```python
from build123d import *

# Parameters (mm, degrees)
BOSS_EXTRUDE1_DEPTH = 3


with BuildPart() as part:
    # Sketch1 → Boss-Extrude1 (new body)
    with BuildSketch(Plane(origin=(0, 0, 0), x_dir=(1, 0, 0), z_dir=(0, 1, 0))):
        with BuildLine():
            Line((0, 0), (3.5, 0))
            Line((3.5, 0), (3.5, 20))
            ThreePointArc((3.5, 20), (9.5, 26), (15.5, 20))
            ThreePointArc((15.5, 20), (17.25, 18.25), (19, 20))
            ThreePointArc((19, 20), (9.5, 29.5), (0, 20))
            Line((0, 20), (0, 0))
        make_face()
    extrude(amount=BOSS_EXTRUDE1_DEPTH)


solid = part.part
```
The model under review builds one solid part; all positions refer to its coordinate system, in mm. Round coordinates to 2 decimals unless told otherwise and drop trailing zeros. Loops run counter-clockwise (first coordinate to the right, second up) from the corner with the lowest first, then second, coordinate; pieces in that order, holes last. Notation, with made-up numbers: M 38,-24 L 49,-24 A26 cw 49,-3 Z; hole C -8.75,15.5 d3. An arc over 180 degrees is marked long. Put each result on its own line as item: value.
Q1. Consider section C-C, the plane x = 9.5. Give the boundary of the cut face in (y, z), then the cut area to 3 significant figures.
Result set:
outline: M 0,-29.5 L 3,-29.5 L 3,-26 L 0,-26 Z
area: 10.5 mm²
Q2. For pin 1 (10 mm diameter, centred on x = 3.5, z = -13, fed in from -Y), flat-tipped, find the tip position at first contact; note if it passes through.
Result set:
pin 1: stops at y = 0
Q3. Mouldability with a two-part tool opening along X and no side actions: class faces 1 (the cylindrical face through (17.21, 1.48, -18.25)), 2 (the cylindrical face through (9.709, 1.479, -29.498)), 3 (the flat face through (3, 3, -18)) as released by +X, released by -X, zero draft, split by the parting line, or undercut.
Result set:
face 1: undercut
face 2: split by the parting line
face 3: zero draft
Q4. Consider section B-B, the plane y = 0.7. Give the boundary of the cut face in (x, z), then the cut area to 3 significant figures.
Result set:
outline: M 0,-20 A9.5 ccw 19,-20 A1.75 ccw 15.5,-20 A6 cw 3.5,-20 L 3.5,0 L 0,0 Z
area: 160 mm²
Q5. Consider section A-A, the plane z = -19.25. Give the boundary of the cut face in (x, y).
Result set:
outline: M 0,0 L 3.5,0 L 3.5,3 L 0,3 Z; M 15.67,0 L 18.83,0 L 18.83,3 L 15.67,3 Z
Q6. Consider section D-D, the plane z = -3.5. Give the boundary of the cut face in (x, y), then the cut area to 3 significant figures.
Result set:
outline: M 0,0 L 3.5,0 L 3.5,3 L 0,3 Z
area: 10.5 mm²
Q7. To check wall thickness, follow L1, parallel to X at y = 2.5, z = -6.5; L2, parallel to X at y = 1.7, z = -22.25; L3, parallel to X at y = 1.4, z = -21.5. State the ranges of each line that lie inside material, in increasing order.
Result set:
L1: x = 0 to 3.5
L2: x = 0.27 to 3.94, 15.06 to 18.73
L3: x = 0.12 to 3.69, 15.31 to 18.88
